Input: part model. Units: mm. Frame: model coordinates. Give positions to 0.01 mm unless a question says otherwise; leave off trailing zeros. Loops run counter-clockwise (first coordinate to the right, second up) from the corner with the lowest first, then second, coordinate; pieces in that order, holes last. Notation, with made-up numbers: M 71,59 L 88,59 A13 ccw 88,83 Z; hole C 63,-35 d7. An arc over 180 degrees is marked long. Use a Markdown table: item, result. Add a question column.
from build123d import *

# Parameters (mm, degrees)
CYLINDER011_R     = 0.8
CYLINDER011_DEPTH = 20
CYLINDER010_R     = 0.8
CYLINDER010_DEPTH = 20
BOX002_W          = 20
BOX002_H          = 10
BOX002_DEPTH      = 10
CYLINDER009_R     = 95
CYLINDER009_DEPTH = 10
FILLET006_R       = 4
FILLET007_R       = 2


with BuildPart() as screw004:
    # Cylinder011 → Cylinder011 (new body)
    with BuildSketch(Plane(origin=(5, -100, 5), x_dir=(1, 0, 0), z_dir=(0, 1, 0))):
        Circle(CYLINDER011_R)
    extrude(amount=CYLINDER011_DEPTH)


with BuildPart() as fusion005:
    # Cylinder010 → Cylinder010 (new body)
    with BuildSketch(Plane(origin=(-5, -100, 5), x_dir=(1, 0, 0), z_dir=(0, 1, 0))):
        Circle(CYLINDER010_R)
    extrude(amount=CYLINDER010_DEPTH)

    # Fusion005: union Screw004
    add(screw004.part)


with BuildPart() as cube001:
    # Box002 → Box002 (new body)
    with BuildSketch(Plane(origin=(-10, -95, 0), x_dir=(1, 0, 0), z_dir=(0, 0, 1))):
        with Locations((10, 5)):
            Rectangle(BOX002_W, BOX002_H)
    extrude(amount=BOX002_DEPTH)


with BuildPart() as obj1:
    # Cylinder009 → Cylinder009 (new body)
    with BuildSketch(Plane.XY):
        Circle(CYLINDER009_R)
    extrude(amount=CYLINDER009_DEPTH)

    # Common: intersect Cube001
    add(cube001.part, mode=Mode.INTERSECT)

    # Fillet006
    fillet006_edges = [obj1.edges().sort_by_distance(p)[0] for p in [
        (-10, -89.736109, 10),
        (10, -89.736109, 10),
    ]]
    fillet(fillet006_edges, radius=FILLET006_R)

    # Fillet007
    fillet007_edges = [obj1.edges().sort_by_distance(p)[0] for p in [
        (0, -85, 10),
    ]]
    fillet(fillet007_edges, radius=FILLET007_R)

    # Cut002: cut Fusion005
    add(fusion005.part, mode=Mode.SUBTRACT)


with BuildPart() as obj1_1:
    # Cut002 placement: moved
    add(obj1.part.moved(Location((0, 0, 2))))


solid = obj1_1.part
1) Ray query, line 1 (X direction, y = -87.75, z = 7); line 2 (Z direction, x = -5, y = -92.75); line 3 (Y direction, x = 0.5, z = 2.5). Return the intervals inside material, ascending. Write a range as [from, to].
2) Section query A-A, the plane y = -89. Return the cut outline in (x, z), and give its area (3 significant figures).
3) Pull-direction query (X, two-part tool) for faces 1 (the cylindrical face through (-8.797, -90.85, 10.859)), 2 (the flat face through (10, -91, 5)), 3 (the cylindrical face through (4.2, -90, 7)); classes: pulls with the +X half, pulls with the -X half, needs draft (parallel to the pull), parting line crosses it, or undercut.
4) Section query D-D, the plane z = 7.5. Return the cut outline in (x, y), and give its area (3 significant figures).
5) Section query C-C, the plane x = -5. Return the cut outline in (y, z).
6) Section query B-B, the plane z = 5.75. Return the cut outline in (x, y), and give its area (3 significant figures).
Entries:
| question | item | result |
|---|---|---|
| 1 | line 1 | x = [-10, -5.8], [-4.2, 4.2], [5.8, 10] |
| 1 | line 2 | z = [2, 6.2], [7.8, 12] |
| 1 | line 3 | y = [-95, -85] |
| 2 | outline | M -10,2 L 10,2 L 10,8 A4 ccw 6,12 L -6,12 A4 ccw -10,8 Z; hole C -5,7 d1.6; hole C 5,7 d1.6 |
| 2 | area | 189 mm² |
| 3 | face 1 | pulls with the -X half |
| 3 | face 2 | pulls with the +X half |
| 3 | face 3 | undercut |
| 4 | outline | M -10,-94.47 A95 ccw -5.62,-94.83 L -5.62,-85 L -8,-85 A2 ccw -10,-87 Z; M -4.38,-94.9 A95 ccw 4.38,-94.9 L 4.38,-85 L -4.38,-85 Z; M 5.62,-94.83 A95 ccw 10,-94.47 L 10,-87 A2 ccw 8,-85 L 5.62,-85 Z |
| 4 | area | 170 mm² |
| 5 | outline | M -94.87,2 L -85,2 L -85,6.2 L -94.87,6.2 Z; M -94.87,7.8 L -85,7.8 L -85,10 A2 ccw -87,12 L -94.87,12 Z |
| 6 | outline | M -10,-94.47 A95 ccw 10,-94.47 L 10,-87 A2 ccw 8,-85 L -8,-85 A2 ccw -10,-87 Z |
| 6 | area | 195 mm² |
